Design review of the part shown in the three views and the two pictorial views. Dimensions are in mm from the part's minimum x, y and z. Give positions to 0.01 mm unless a question says otherwise; leave off trailing zeros. Write each loop counter-clockwise with the first axis right and the second up, starting at its lowest first coordinate (ties: lowest second). Pieces come first, ordered by that corner, then holes.
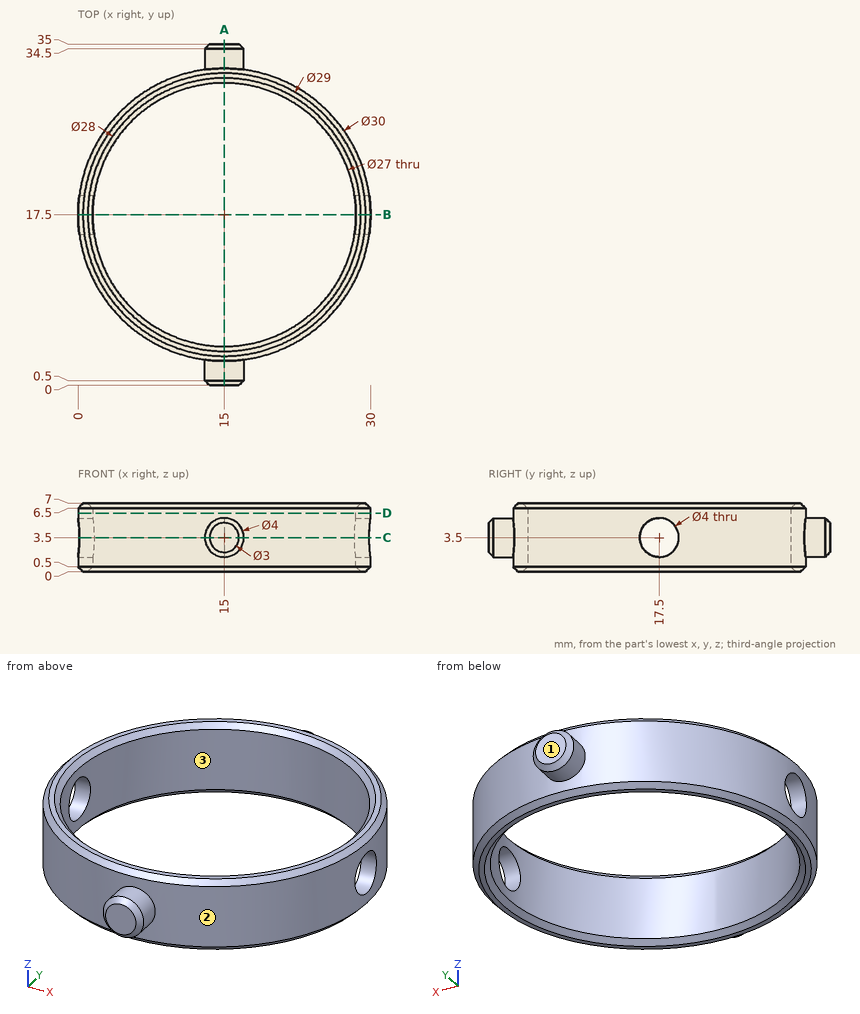
(1) Consider section B-B, the plane y = 17.5. Give the boundary of the cut face in (x, z), then the cut area to 3 significant figures.
Resolved:
outline: (0, 0.5) - (0.5, 0) - (1, 0) - (1.5, 0.5) - (1.5, 1.5) - (0, 1.5) - close; (0, 5.5) - (1.5, 5.5) - (1.5, 6.5) - (1, 7) - (0.5, 7) - (0, 6.5) - close; (28.5, 0.5) - (29, 0) - (29.5, 0) - (30, 0.5) - (30, 1.5) - (28.5, 1.5) - close; (28.5, 5.5) - (30, 5.5) - (30, 6.5) - (29.5, 7) - (29, 7) - (28.5, 6.5) - close
area: 8.00 mm2
(2) Consider section C-C, the plane z = 3.5. Give the boundary of the cut face in (x, y), then the cut area to 3 significant figures.
Resolved:
outline: (0.13, 15.5) arc R15 ccw to (13, 2.63) - (13, 0.5) - (13.5, 0) - (16.5, 0) - (17, 0.5) - (17, 2.63) arc R15 ccw to (29.87, 15.5) - (28.35, 15.5) arc R13.5 cw to (1.65, 15.5) - close; (0.13, 19.5) - (1.65, 19.5) arc R13.5 cw to (28.35, 19.5) - (29.87, 19.5) arc R15 ccw to (17, 32.37) - (17, 34.5) - (16.5, 35) - (13.5, 35) - (13, 34.5) - (13, 32.37) arc R15 ccw to start
area: 142 mm2
(3) To check wall thickness, follow L1, parallel to X at y = 18, z = 1.25; L2, parallel to Y at x = 16, z = 4.75; L3, parallel to X at y = 11.5, z = 1. State the ranges of each line that lie inside material, in increasing order.
Resolved:
L1: x = 0.01 to 1.51, 28.49 to 29.99
L2: y = 0.1 to 4.04, 30.96 to 34.9
L3: x = 1.25 to 2.91, 27.09 to 28.75
(4) Consider section D-D, the plane z = 6. Give the boundary of the cut face in (x, y), then the cut area to 3 significant figures.
Resolved:
outline: circle Ø30 at (15, 17.5); hole circle Ø27 at (15, 17.5)
area: 134 mm2
(5) Mouldability with a two-part tool opening along Y and no side actions: class the marked faces 1, 2 and 3 as pulls with the +Y half, pulls with the -Y half, needs draft (parallel to the pull), parting line crosses it, or undercut.
Resolved:
face 1: pulls with the +Y half
face 2: parting line crosses it
face 3: undercut
(6) Clearance check with flat-ended pins moving along their axes: P1, Ø1, axis at y = 13, z = 4.5, coming from the +X side; P2, Ø4, axis at y = 12.5, z = 1.5, coming from the +X side; P3, Ø2, axis at x = 26.5, z = 5, coming from the -Y side; P4, Ø10, axis at x = 8, y = 25, coming from the +Z side. State where each tip first meets the part, or that it passes through.
Resolved:
P1: stops at x = 29.46
P2: stops at x = 29.7
P3: stops at y = 6.79
P4: stops at z = 7
(7) Consider section A-A, the plane x = 15. Give the boundary of the cut face in (y, z).
Resolved:
outline: (0, 2) - (0.5, 1.5) - (2.5, 1.5) - (2.5, 0.5) - (3, 0) - (3.5, 0) - (4, 0.5) - (4, 6.5) - (3.5, 7) - (3, 7) - (2.5, 6.5) - (2.5, 5.5) - (0.5, 5.5) - (0, 5) - close; (31, 0.5) - (31.5, 0) - (32, 0) - (32.5, 0.5) - (32.5, 1.5) - (34.5, 1.5) - (35, 2) - (35, 5) - (34.5, 5.5) - (32.5, 5.5) - (32.5, 6.5) - (32, 7) - (31.5, 7) - (31, 6.5) - close
